CAD build for the part. Positions are in the model's coordinates, mm. Face numbers are marked on the shaded views. A direction names the side the tool comes from. Give positions to 0.01 mm unless a question says otherwise; leave off trailing zeros. Loops run counter-clockwise (first coordinate to the right, second up) from the corner with the lowest first, then second, coordinate; pieces in that order, holes last. Notation, with made-up numbers: (-6, 6.5) - (52, 6.5) arc R33 cw to (52, 43.5) - close; hole circle Ø3 at (-31, 45). An arc over 180 degrees is marked (long way). Return JSON: item names as keys, results as strings.
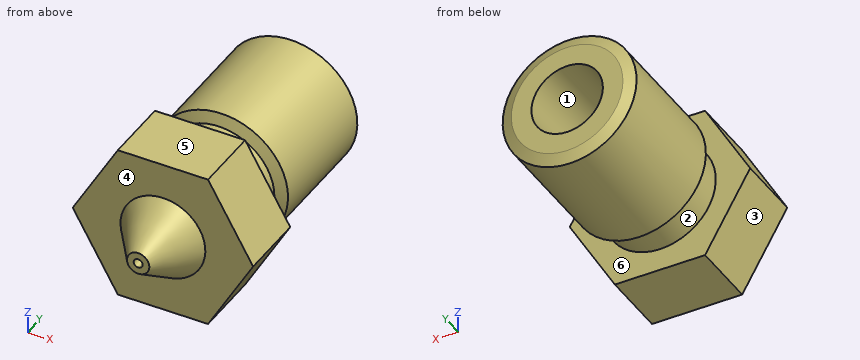
from build123d import *

# Parameters (mm, degrees)
BOSS_EXTRUDE1_DEPTH = 3


with BuildPart() as part:
    # Sketch1 → Revolve1 (revolve)
    with BuildSketch(Plane.XY, mode=Mode.PRIVATE) as revolve1_sk:
        Polygon((0, 0), (0.5, 0), (1.900415076, 2), (3.5, 2), (3.5, 5), (2.5, 5), (2.5, 6.5), (3, 6.7), (3, 12.3), (2.5, 12.5), (0, 12.5), align=None)
    revolve(revolve1_sk.sketch.rotate(Axis((0, 0, 0), (0, 1, 0)), 90), axis=Axis((0, 0, 0), (0, 1, 0)))

    # Sketch2 → Boss-Extrude1 (add)
    with BuildSketch(Plane(origin=(0, 5, 0), x_dir=(1, 0, 0), z_dir=(0, 1, 0))):
        Polygon((2.020725942, 3.5), (-2.020725942, 3.5), (-4.041451884, 0), (-2.020725942, -3.5), (2.020725942, -3.5), (4.041451884, 0), align=None)
    extrude(amount=-BOSS_EXTRUDE1_DEPTH)

    # Sketch3 → Cut-Revolve1 (revolve, cut)
    with BuildSketch(Plane.XY, mode=Mode.PRIVATE) as cut_revolve1_sk:
        Polygon((0, 0), (0.2, 0), (0.2, 0.8), (0.75, 1.117542648), (0.75, 1.909252271), (1.6, 2.4), (1.6, 12.5), (0, 12.5), align=None)
    revolve(cut_revolve1_sk.sketch.rotate(Axis((0, 0, 0), (0, 1, 0)), 90), axis=Axis((0, 0, 0), (0, 1, 0)), mode=Mode.SUBTRACT)


solid = part.part
1. Which spindle directions (+Z, -Z, +X, -X, +Y, -Y) get a long thin tool onto all of the face, cutting with end or side? Do the marked faces 1, 2 and 3. Say none if no direction does.
Values follow:
{"face 1": "+Y", "face 2": "none", "face 3": "-Z, -X, +Y, -Y"}
2. Pull direction Y, two halves, no side cores. Call the marked faces 4, 5 and 6: +Y half, -Y half, draft (parallel to the pull), parting line (faces both ways), or undercut.
Values follow:
{"face 4": "-Y half", "face 5": "draft", "face 6": "undercut"}
3. Cut at D-D, the plane z = 3.25. Write the cut outline in (x, y), plus the area to 3 significant figures.
Values follow:
{"outline": "(-2.17, 2) - (2.17, 2) - (2.17, 5) - (-2.17, 5) - close", "area": "13.0 mm²"}
4. Drill centre lines: probe 1 along X at (y, z) = (8.5, 0); probe 2 along Y at (x, z) = (3.25, -0.75); probe 3 along X at (y, z) = (7.5, 1). Where is each one in solid material? Low to high.
Values follow:
{"probe 1": "x = -3 to -1.6, 1.6 to 3", "probe 2": "y = 2 to 5", "probe 3": "x = -2.83 to -1.25, 1.25 to 2.83"}
5. Drop flat-ended pins along their axis: P1, Ø1.5, axis at x = -3, z = 0, coming from the -Y side; P2, Ø3, axis at x = 0.5, y = 8.5, coming from the +Z side; P3, Ø0.9, axis at x = 0, z = 0, coming from the +Y side. Give the stop position or say it passes through.
Values follow:
{"P1": "stops at y = 2", "P2": "stops at z = 3", "P3": "stops at y = 0.94"}
6. Cut at C-C, the plane y = 7.5. Write the cut outline in (x, z).
Values follow:
{"outline": "circle Ø6 at (0, 0); hole circle Ø3.2 at (0, 0)"}
7. Cut at B-B, the plane y = 6.25. Write the cut outline in (x, z), plus the area to 3 significant figures.
Values follow:
{"outline": "circle Ø5 at (0, 0); hole circle Ø3.2 at (0, 0)", "area": "11.6 mm²"}
